```python
from build123d import *

# Parameters (mm, degrees)
SKETCH1_R               = 1.2065
SKETCH1_R_2             = 1.0795
BOSS_EXTRUDE1_DEPTH     = 10
SKETCH2_W               = 4.648816228
SKETCH2_H               = 2.032
CUT_EXTRUDE1_DEPTH      = 1.5
CUT_EXTRUDE2_DEPTH      = 5
CUT_EXTRUDE2_DEPTH_BACK = 5
SKETCH4_R               = 0.1984375


with BuildPart() as part:
    # Sketch1 → Boss-Extrude1 (new body)
    with BuildSketch(Plane(origin=(0, 0, 0), x_dir=(0, 0, -1), z_dir=(1, 0, 0))):
        Circle(SKETCH1_R)
        Circle(SKETCH1_R_2, mode=Mode.SUBTRACT)
    extrude(amount=BOSS_EXTRUDE1_DEPTH)

    # Sketch2 → Cut-Extrude1 (cut)
    with BuildSketch(Plane.ZY):
        with Locations((0.126795446, 0)):
            Rectangle(SKETCH2_W, SKETCH2_H)
    extrude(amount=-CUT_EXTRUDE1_DEPTH, mode=Mode.SUBTRACT)

    # Sketch4 → Cut-Extrude2 (cut, two sides: drawn at the far end of the back side and taken through both)
    with BuildSketch(Plane(origin=(0, 0, 0), x_dir=(1, 0, 0), z_dir=(0, 1, 0)).offset(-CUT_EXTRUDE2_DEPTH_BACK)):
        with Locations(Location((1, 0, 0), (0, 0, 90))):
            Circle(SKETCH4_R)
    extrude(amount=CUT_EXTRUDE2_DEPTH + CUT_EXTRUDE2_DEPTH_BACK, mode=Mode.SUBTRACT)


solid = part.part
```
Design review of the part built by this model. Coordinates are the model's own, in mm. Give positions to 0.01 mm unless a question says otherwise; leave off trailing zeros. Order: outer loops, then holes, each group sorted by start corner. A loop starts at its lowest first (then second) coordinate and runs counter-clockwise, first axis right, second up. Notation, with made-up numbers: (-6, 27.25) -> (37, 27.25) arc R17 cw to (37, 58.25) -> close; hole circle Ø3 at (67.25, -3.5). An arc over 180 degrees is marked (long way). Write item = value, one per line. Start each with the question number.
(1) We need section D-D on x = 7.25. Write out the cut boundary in (y, z).
(2) To check wall thickness, follow line 1 along X through (y, z) = (-1.15, 0); line 2 along X through (y, z) = (0.65, 0.9); line 3 along Z through (x, y) = (1, -1.1). State the ranges of each line that lie inside material, in increasing order.
(3) We need section B-B on y = 0. Write out the cut boundary in (x, z), plus the area to 3 significant figures.
(4) We need section C-C on x = 1. Write out the cut boundary in (y, z), plus the area to 3 significant figures.
(5) We need section A-A on z = 0. Write out the cut boundary in (x, y).
Numbers:
q1.outline = circle Ø2.41 at (0, 0); hole circle Ø2.16 at (0, 0)
q2.line_1 = 0 to 0.8, 1.2 to 10
q2.line_2 = 1.5 to 10
q2.line_3 = -0.5 to -0.2, 0.2 to 0.5
q3.outline = (1.5, -1.21) -> (10, -1.21) -> (10, -1.08) -> (1.5, -1.08) -> close; (1.5, 1.08) -> (10, 1.08) -> (10, 1.21) -> (1.5, 1.21) -> close
q3.area = 2.16 mm^2
q4.outline = (-1.19, -0.2) arc R1.21 ccw to (-1.02, -0.65) -> (-1.02, -0.36) arc R1.08 cw to (-1.06, -0.2) -> close; (-1.19, 0.2) -> (-1.06, 0.2) arc R1.08 cw to (-1.02, 0.36) -> (-1.02, 0.65) arc R1.21 ccw to start; (1.02, -0.65) arc R1.21 ccw to (1.19, -0.2) -> (1.06, -0.2) arc R1.08 cw to (1.02, -0.36) -> close; (1.02, 0.36) arc R1.08 cw to (1.06, 0.2) -> (1.19, 0.2) arc R1.21 ccw to (1.02, 0.65) -> close
q4.area = 0.173 mm^2
q5.outline = (0, -1.21) -> (0.8, -1.21) -> (0.8, -1.08) -> (0, -1.08) -> close; (0, 1.08) -> (0.8, 1.08) -> (0.8, 1.21) -> (0, 1.21) -> close; (1.2, -1.21) -> (10, -1.21) -> (10, -1.08) -> (1.2, -1.08) -> close; (1.2, 1.08) -> (10, 1.08) -> (10, 1.21) -> (1.2, 1.21) -> close
